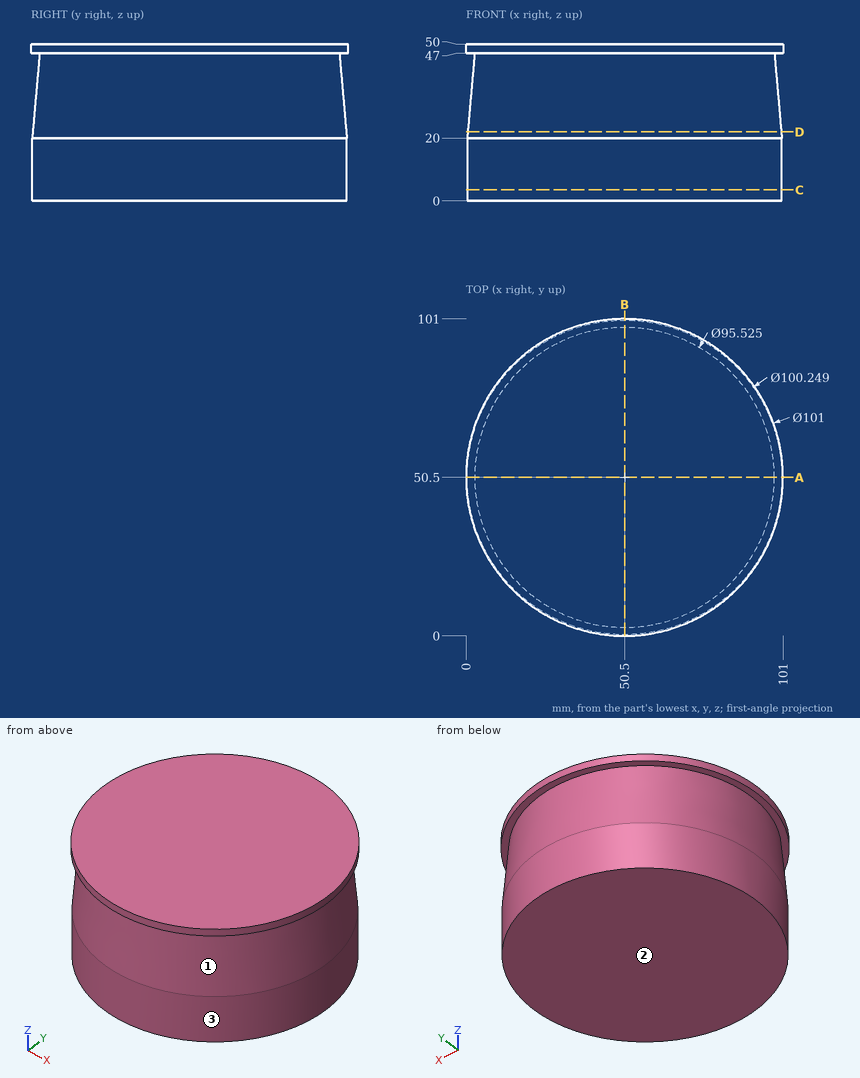
Verification items for this drawing (mm, ordinates from the low corner). Round coordinates to 2 decimals unless told otherwise and drop trailing zeros. Loops run counter-clockwise (first coordinate to the right, second up) from the corner with the lowest first, then second, coordinate; pieces in that order, holes last. Notation, with made-up numbers: (51, 71) - (105, 71) arc R12 ccw to (105, 93) - close; hole circle Ø2 at (52.25, -4.75). An arc over 180 degrees is marked (long way). Write item = value, one per line.
Q1. Sectioned sample at D-D on z = 22. Record the boundary of the cut face in (x, y).
Here are the results:
outline = circle Ø99.9 at (50.5, 50.5)
Q2. Material ranges on L1, parallel to Y at x = 49, z = 7; L2, parallel to X at y = 88.5, z = 30; L3, parallel to Y at x = 64, z = 40, recorded low to high.
Here are the results:
L1 = 0.4 to 100.6
L2 = 19.17 to 81.83
L3 = 4.05 to 96.95
Q3. Sectioned sample at A-A on y = 50.5. Record the boundary of the cut face in (x, z) (1 decimal), plus the area to 3 significant figures.
Here are the results:
outline = (0, 47) - (2.7, 47) - (0.4, 20) - (0.4, 0) - (100.6, 0) - (100.6, 20) - (98.3, 47) - (101, 47) - (101, 50) - (0, 50) - close
area = 4,950 mm^2
Q4. Mould release check, pull along Z, two halves, no side actions. Record for the marked faces 1, 2 and 3: +Z half, -Z half, draft (parallel to the pull), parting line (faces both ways), or undercut.
Here are the results:
face_1 = undercut
face_2 = -Z half
face_3 = draft
Q5. Depth check by flat-ended pin: pin 1 (1 mm diameter, centred on y = 40.5, z = 20.5, fed in from +X); pin 2 (12 mm diameter, centred on x = 41.5, y = 70, fed in from -Z); pin 3 (5 mm diameter, centred on y = 57, z = 14, fed in from +X) (1 decimal); pin 4 (4 mm diameter, centred on y = 23.5, z = 29, fed in from -X). Enter the tip coordinate at first touch or a pass-through.
Here are the results:
pin_1 = 99.68
pin_2 = 0
pin_3 = 100.5
pin_4 = 7.95
Q6. Sectioned sample at C-C on z = 3.5. Record the boundary of the cut face in (x, y) (1 decimal).
Here are the results:
outline = circle Ø100.2 at (50.5, 50.5)
